from build123d import *

# Parameters (mm, degrees)
EXTRU_MINCE1_DEPTH      = 10
BOSS_EXTRU_1_DEPTH      = 2
ESQUISSE2_OUTSIDE_W     = 106.586
ESQUISSE2_OUTSIDE_H     = 101.586
ENL_V_MAT_EXTRU_1_DEPTH = 3
ESQUISSE3_R             = 3.9
BOSS_EXTRU_2_DEPTH      = 23
ESQUISSE9_R             = 1.5
ENL_V_MAT_EXTRU_2_DEPTH = 1.5
ESQUISSE12_R            = 1.5
ENL_V_MAT_EXTRU_3_DEPTH = 21


with BuildPart() as part:
    # Esquisse1 → Extru.-Mince1 (new body)
    with BuildSketch(Plane.XY):
        with BuildLine():
            Line((37.5, -38.5), (-37.5, -38.5))
            ThreePointArc((-37.5, -38.5), (-39.974873734, -37.474873734), (-41, -35))
            Line((-41, -35), (-41, 35))
            ThreePointArc((-41, 35), (-39.974873734, 37.474873734), (-37.5, 38.5))
            Line((-37.5, 38.5), (37.5, 38.5))
            ThreePointArc((37.5, 38.5), (39.974873734, 37.474873734), (41, 35))
            Line((41, 35), (41, -35))
            ThreePointArc((41, -35), (39.974873734, -37.474873734), (37.5, -38.5))
        make_face()
        with BuildLine():
            Line((37.5, -36.5), (-37.5, -36.5))
            ThreePointArc((-37.5, -36.5), (-38.560660172, -36.060660172), (-39, -35))
            Line((-39, -35), (-39, 35))
            ThreePointArc((-39, 35), (-38.560660172, 36.060660172), (-37.5, 36.5))
            Line((-37.5, 36.5), (37.5, 36.5))
            ThreePointArc((37.5, 36.5), (38.560660172, 36.060660172), (39, 35))
            Line((39, 35), (39, -35))
            ThreePointArc((39, -35), (38.560660172, -36.060660172), (37.5, -36.5))
        make_face(mode=Mode.SUBTRACT)
    extrude(amount=EXTRU_MINCE1_DEPTH)

    # Esquisse1<2> → Boss.-Extru.1 (add)
    with BuildSketch(Plane.XY):
        with BuildLine():
            Line((-37.5, 37.5), (37.5, 37.5))
            ThreePointArc((37.5, 37.5), (39.267766953, 36.767766953), (40, 35))
            Line((40, 35), (40, -35))
            ThreePointArc((40, -35), (39.267766953, -36.767766953), (37.5, -37.5))
            Line((37.5, -37.5), (-37.5, -37.5))
            ThreePointArc((-37.5, -37.5), (-39.267766953, -36.767766953), (-40, -35))
            Line((-40, -35), (-40, 35))
            ThreePointArc((-40, 35), (-39.267766953, 36.767766953), (-37.5, 37.5))
        make_face()
    extrude(amount=BOSS_EXTRU_1_DEPTH)

    # Esquisse2 outside → Enlèv. mat.-Extru.1 (cut)
    with BuildSketch(Plane.XY.offset(10)):
        Rectangle(ESQUISSE2_OUTSIDE_W, ESQUISSE2_OUTSIDE_H)
        with BuildLine():
            Line((-37.5, 37.5), (37.5, 37.5))
            ThreePointArc((37.5, 37.5), (39.267766953, 36.767766953), (40, 35))
            Line((40, 35), (40, -35))
            ThreePointArc((40, -35), (39.267766953, -36.767766953), (37.5, -37.5))
            Line((37.5, -37.5), (-37.5, -37.5))
            ThreePointArc((-37.5, -37.5), (-39.267766953, -36.767766953), (-40, -35))
            Line((-40, -35), (-40, 35))
            ThreePointArc((-40, 35), (-39.267766953, 36.767766953), (-37.5, 37.5))
        make_face(mode=Mode.SUBTRACT)
    extrude(amount=-ENL_V_MAT_EXTRU_1_DEPTH, mode=Mode.SUBTRACT)

    # Esquisse3 → Boss.-Extru.2 (add)
    with BuildSketch(Plane.XY.offset(2)):
        with Locations((-25.2, 27.7)):
            Circle(ESQUISSE3_R)
        with Locations((25.2, 27.7)):
            Circle(ESQUISSE3_R)
        with Locations((-25.2, -27.7)):
            Circle(ESQUISSE3_R)
        with Locations((25.2, -27.7)):
            Circle(ESQUISSE3_R)
    extrude(amount=BOSS_EXTRU_2_DEPTH)

    # Esquisse9 → Enlèv. mat.-Extru.2 (cut)
    with BuildSketch(Plane.XY.offset(25)):
        with Locations((-25.2, 27.7)):
            Circle(ESQUISSE9_R)
        with Locations((25.2, 27.7)):
            Circle(ESQUISSE9_R)
        with Locations((-25.2, -27.7)):
            Circle(ESQUISSE9_R)
        with Locations((25.2, -27.7)):
            Circle(ESQUISSE9_R)
    extrude(amount=-ENL_V_MAT_EXTRU_2_DEPTH, mode=Mode.SUBTRACT)

    # Esquisse12 → Enlèv. mat.-Extru.3 (cut)
    with BuildSketch(Plane(origin=(0, 0, 0), x_dir=(-1, 0, 0), z_dir=(0, 0, -1))):
        with Locations((24.9, 27.4)):
            Circle(ESQUISSE12_R)
        with Locations((-24.9, 27.4)):
            Circle(ESQUISSE12_R)
        with Locations((-24.9, -27.4)):
            Circle(ESQUISSE12_R)
        with Locations((24.9, -27.4)):
            Circle(ESQUISSE12_R)
    extrude(amount=-ENL_V_MAT_EXTRU_3_DEPTH, mode=Mode.SUBTRACT)


solid = part.part
Model file for the job. Use its own axes, mm. A direction names the side the tool comes from. Give positions to 0.01 mm unless a question says otherwise; leave off trailing zeros. Loops run counter-clockwise (first coordinate to the right, second up) from the corner with the lowest first, then second, coordinate; pieces in that order, holes last.
1) Wall check: line 1 (Y direction, x = 24.9, z = 16.5); line 2 (Y direction, x = 24.9, z = 9.5); line 3 (Y direction, x = 25.2, z = 24.6). Give the ranges that are in metal, low to high.
2) Saw through at C-C (x = 5). Write the cut outline in (y, z), plus the area to 3 significant figures.
3) Tool access for faces 4 (the flat face through (-25, -27, 21)), 5 (the cylindrical face through (24.09, -26.69, 24.26)), 6 (the cylindrical face through (-39, -37, 9)): list every direction of +Z, -Z, +X, -X, +Y, -Y with a clear straight run to the whole face (end or side of a thin tool).
4) Saw through at D-D (y = 1.5). Write the cut outline in (x, z), plus the area to 3 significant figures.
5) Pull direction Y, two halves, no side cores. Call faces 1 (the cylindrical face through (24.355, -31.507, 13.339)), 2 (the flat face through (-1, 38.5, 3)), 3 (the flat face through (1, -37.5, 9)): +Y half, -Y half, draft (parallel to the pull), parting line (faces both ways), or undercut.
6) Saw through at B-B (z = 5). Count the separate pieces of the cut face and the enclosed holes in it, plus the area to 3 significant figures.
7) Flat gauge pins, fed straight in: pin 1 Ø10 at (x, y) = (12.5, 9) entering from +Z; pin 2 Ø2.5 at (y, z) = (-5, 9) entering from -X; pin 3 Ø12 at (x, z) = (11, 13.5) entering from -Y. Where does each tip first touch, or does it go through?
8) Saw through at A-A (z = 16.5). Write the cut outline in (x, y), plus the area to 3 significant figures.
Answer block:
1. line 1: y = -31.59 to -28.9, -25.9 to -23.81, 23.81 to 25.9, 28.9 to 31.59
1. line 2: y = -37.5 to -36.5, -31.59 to -28.9, -25.9 to -23.81, 23.81 to 25.9, 28.9 to 31.59, 36.5 to 37.5
1. line 3: y = -31.6 to -29.2, -26.2 to -23.8, 23.8 to 26.2, 29.2 to 31.6
2. outline: (-38.5, 0) - (38.5, 0) - (38.5, 7) - (37.5, 7) - (37.5, 10) - (36.5, 10) - (36.5, 2) - (-36.5, 2) - (-36.5, 10) - (-37.5, 10) - (-37.5, 7) - (-38.5, 7) - close
2. area: 180 mm2
3. face 4: -Z
3. face 5: +Z
3. face 6: +Z, -X, -Y
4. outline: (-41, 0) - (41, 0) - (41, 7) - (40, 7) - (40, 10) - (39, 10) - (39, 2) - (-39, 2) - (-39, 10) - (-40, 10) - (-40, 7) - (-41, 7) - close
4. area: 190 mm2
5. face 1: undercut
5. face 2: +Y half
5. face 3: -Y half
6. separate pieces: 5
6. enclosed holes: 5
6. area: 774 mm2
7. pin 1: stops at z = 2
7. pin 2: stops at x = -40
7. pin 3: stops at y = -37.5
8. outline: circle Ø7.8 at (-25.2, -27.7); circle Ø7.8 at (-25.2, 27.7); circle Ø7.8 at (25.2, -27.7); circle Ø7.8 at (25.2, 27.7); hole circle Ø3 at (-24.9, -27.4); hole circle Ø3 at (-24.9, 27.4); hole circle Ø3 at (24.9, -27.4); hole circle Ø3 at (24.9, 27.4)
8. area: 163 mm2
